```python
from build123d import *

# Parameters (mm, degrees)
F0_W      = 114
F0_H      = 49
F0_W_2    = 86
F0_H_2    = 8
F1_DEPTH  = 3
F0_W_3    = 120
F0_H_3    = 55
F2_DEPTH  = 47
F3_R      = 3
F4_DEPTH  = 130
F5_R      = 3
F6_DEPTH  = 10
F7_W      = 5
F7_H      = 20
F8_DEPTH  = 120
F9_R      = 3
F10_DEPTH = 25
F11_R     = 10
F12_R     = 2.99999


# Not quite as in the source:
# - a fillet or chamfer is up to 0.001 mm smaller than in the source, because OpenCascade refuses the exact size


with BuildPart() as f1:
    # F0 (on Top) → F1 (new body)
    with BuildSketch(Plane.XY):
        with Locations((60, 27.5)):
            Rectangle(F0_W, F0_H)
        with Locations((66, 21)):
            Rectangle(F0_W_2, F0_H_2, mode=Mode.SUBTRACT)
    extrude(amount=-F1_DEPTH)

    # F0 (on Top) → F2 (join)
    with BuildSketch(Plane.XY):
        with Locations((60, 27.5)):
            Rectangle(F0_W_3, F0_H_3)
        with Locations((60, 27.5)):
            Rectangle(F0_W, F0_H, mode=Mode.SUBTRACT)
    extrude(amount=-F2_DEPTH)

    # F3 (on Right) → F4 (cut)
    with BuildSketch(Plane.YZ):
        with Locations((39, -36)):
            Circle(F3_R)
        with Locations((16, -36)):
            Circle(F3_R)
    extrude(amount=F4_DEPTH, mode=Mode.SUBTRACT)

    # F5 (on Front) → F6 (cut)
    with BuildSketch(Plane.XZ):
        with Locations((35, -33)):
            Circle(F5_R)
        with Locations((85, -33)):
            Circle(F5_R)
    extrude(amount=-F6_DEPTH, mode=Mode.SUBTRACT)

    # F7 (on Right) → F8 (join)
    with BuildSketch(Plane.YZ):
        with Locations((2.5, 10)):
            Rectangle(F7_W, F7_H)
    extrude(amount=F8_DEPTH)

    # F9 (on Front) → F10 (cut)
    with BuildSketch(Plane.XZ):
        with Locations((15, 10)):
            Circle(F9_R)
        with Locations((60, 10)):
            Circle(F9_R)
        with Locations((105, 10)):
            Circle(F9_R)
    extrude(amount=-F10_DEPTH, mode=Mode.SUBTRACT)

    # F11
    f11_edges = [f1.edges().sort_by_distance(p)[0] for p in [
        (0, 2.5, 20),
        (120, 2.5, 20),
    ]]
    fillet(f11_edges, radius=F11_R)

    # F12 (radius 3 in the source; OpenCascade refuses exactly that, so slightly less here)
    f12_edges = [f1.edges().sort_by_distance(p)[0] for p in [
        (66, 17, 0),
        (60, 55, 0),
        (120, 30, 0),
        (60, 5, 0),
        (0, 30, 0),
        (109, 21, 0),
        (66, 25, 0),
        (23, 21, 0),
        (120, 55, -23.5),
        (0, 55, -23.5),
        (2.928932, 5, 17.071068),
        (60, 5, 20),
        (117.071068, 5, 17.071068),
    ]]
    fillet(f12_edges, radius=F12_R)


solid = f1.part
```
Check sheet for the modelled part. Datum: model origin and axes. Units: mm. A direction names the side the tool comes from. Give positions to 0.01 mm unless a question says otherwise; leave off trailing zeros. Write each loop counter-clockwise with the first axis right and the second up, starting at its lowest first coordinate (ties: lowest second). Pieces come first, ordered by that corner, then holes.
Item 1: Cross-section at C-C (x = 15). Enter the section's corners in (y, z), and give its area (3 significant figures).
Item 2: Cross-section at D-D (y = 39). Enter the section's corners in (x, z), and give its area (3 significant figures).
Item 3: Cross-section at B-B (z = -15). Enter the section's corners in (x, y), and give its area (3 significant figures).
Item 4: Draft check along Z on faces 1 (the face through (59, 55, -25)), 2 (the face through (118.48, 13.79, -33.97)), 3 (the face through (60.8, 5.86, 0.9)), 4 (the face through (59, 28, -3)). Enter one of: released by +Z, released by -Z, zero draft, split by the parting line, or undercut.
Item 5: Access from +Z, -Z, +X, -X, +Y, -Y to the whole of each face (thin tool, end or side, straight path). Record for faces 5 (the face through (66.64, 25.9, -0.86)), 6 (the face through (119.14, 4.1, 6.55)), 7 (the face through (69, 54, -47)), 8 (the face through (59, 3, -25)).
Item 6: Gauge pin test, flat ends, axial feed: pin 1 (5.5 mm diameter, centred on y = 39, z = -36, fed in from +X); pin 2 (1 mm diameter, centred on x = 38, z = -24.5, fed in from -Y); pin 3 (6 mm diameter, centred on x = 18, y = 32.5, fed in from +Z); pin 4 (14.5 mm diameter, centred on x = 63, y = 23, fed in from -Z). Record the tip position at first contact, or that the pin passes through.
Item 7: Scan lines: L1, parallel to Y at x = 47.5, z = -23.5; L2, parallel to X at y = 44, z = -22.5; L3, parallel to Y at x = 117.7, z = -36. Record each from-to range of solid material in increasing order.
Item 8: Cross-section at A-A (x = 60). Count the separate pieces of the cut face and the enclosed holes in it, and give its area (3 significant figures).
Report:
1. outline: (0, -47) - (3, -47) - (3, -3) - (52, -3) - (52, -47) - (55, -47) - (55, -3) arc R3 ccw to (52, 0) - (8, 0) arc R3 cw to (5, 3) - (5, 7) - (0, 7) - close; (0, 13) - (5, 13) - (5, 17) arc R3 ccw to (2, 20) - (0, 20) - close
1. area: 497 mm2
2. outline: (0, -47) - (3, -47) - (3, -39) - (0, -39) - close; (0, -33) - (3, -33) - (3, -3) - (117, -3) - (117, -33) - (120, -33) - (120, -3) arc R3 ccw to (117, 0) - (3, 0) arc R3 ccw to (0, -3) - close; (117, -47) - (120, -47) - (120, -39) - (117, -39) - close
2. area: 584 mm2
3. outline: (0, 0) - (120, 0) - (120, 52) arc R3 ccw to (117, 55) - (3, 55) arc R3 ccw to (0, 52) - close; hole (3, 3) - (117, 3) - (117, 52) - (3, 52) - close
3. area: 1,010 mm2
4. face 1: zero draft
4. face 2: undercut
4. face 3: released by +Z
4. face 4: released by -Z
5. face 5: +Z
5. face 6: +Z, +X, +Y
5. face 7: -Z, +X, -X, +Y, -Y
5. face 8: -Z
6. pin 1: passes through
6. pin 2: stops at y = 0
6. pin 3: stops at z = 0
6. pin 4: stops at z = -3
7. L1: y = 0 to 3, 52 to 55
7. L2: x = 0 to 3, 117 to 120
7. L3: y = 0 to 13, 19 to 36, 42 to 54.92
8. separate pieces: 3
8. enclosed holes: 0
8. area: 469 mm2
